Source: CAD feature listing. Evaluate the final solid. Frame: model axes, mm. Face numbers are marked on the shaded views. A direction names the side the tool comes from. Give positions to 0.01 mm unless a question says otherwise; leave off trailing zeros. Order: outer loops, then holes, each group sorted by start corner. A loop starts at its lowest first (then second) coordinate and runs counter-clockwise, first axis right, second up. Notation, with made-up numbers: (7.5, 28.25) -> (56.5, 28.25) arc R34 cw to (56.5, 60.25) -> close; hole circle Ø6 at (-23, -35). An arc over 180 degrees is marked (long way). Answer in a Markdown table with one row per item.
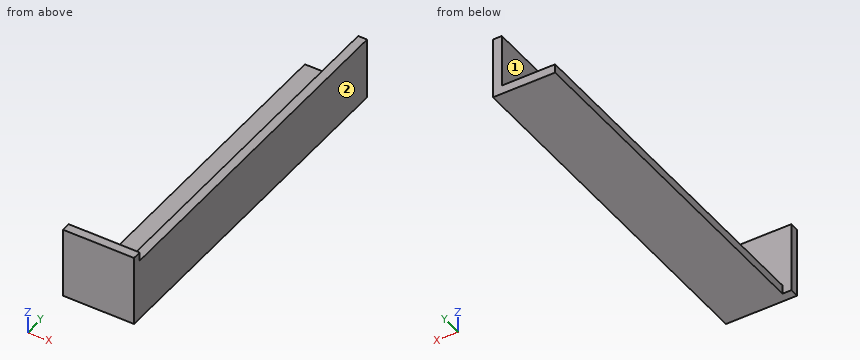
```python
from build123d import *

# Parameters (mm, degrees)
SKETCH_1_W           = 100
SKETCH_1_H           = 100
EXTRUDE_1_DEPTH      = 10
EXTRUDE_2_DEPTH      = 400
SKETCH_3_OUTSIDE_W   = 188.74
SKETCH_3_OUTSIDE_H   = 188.74
SKETCH_3_OUTSIDE_W_2 = 80
SKETCH_3_OUTSIDE_H_2 = 80
CUT_EXTRUDE_1_DEPTH  = 400


with BuildPart() as part:
    # 草图1 → 凸台-拉伸1 (new body)
    with BuildSketch(Plane(origin=(0, 0, 0), x_dir=(1, 0, 0), z_dir=(0, 1, 0))):
        with Locations((11.323542268, -6.987712791)):
            Rectangle(SKETCH_1_W, SKETCH_1_H)
    extrude(amount=EXTRUDE_1_DEPTH)

    # 草图2 → 凸台-拉伸2 (add)
    with BuildSketch(Plane(origin=(0, 10, 0), x_dir=(1, 0, 0), z_dir=(0, 1, 0))):
        Polygon((51.323542268, 33.012287209), (-18.676457732, 33.012287209), (-18.676457732, 23.012287209), (41.323542268, 23.012287209), (41.323542268, -36.987712791), (51.323542268, -36.987712791), align=None)
    extrude(amount=EXTRUDE_2_DEPTH)

    # 草图3 outside → 切除-拉伸1 (cut)
    with BuildSketch(Plane(origin=(0, 10, 0), x_dir=(1, 0, 0), z_dir=(0, 1, 0))):
        with Locations((11.324, -6.988)):
            Rectangle(SKETCH_3_OUTSIDE_W, SKETCH_3_OUTSIDE_H)
        with Locations((11.323542268, -6.987712791)):
            Rectangle(SKETCH_3_OUTSIDE_W_2, SKETCH_3_OUTSIDE_H_2, mode=Mode.SUBTRACT)
    extrude(amount=-CUT_EXTRUDE_1_DEPTH, mode=Mode.SUBTRACT)


solid = part.part
```
(1) Access query for the marked faces 1 and 2. Directions: +Z, -Z, +X, -X, +Y, -Y. A direction counts if a zero-diameter tool reaches every point of the face in a straight line with its end or side. Return the directions, or none.
A:
| item | result |
|---|---|
| face 1 | +Z, -X, +Y |
| face 2 | +Z, -Z, +X, +Y, -Y |
(2) First-contact query: pin 1 Ø5 at (x, y) = (13.5, 216.5) entering from +Z; pin 2 Ø1 at (x, z) = (-2, 14) entering from +Y; pin 3 Ø3 at (x, y) = (47.5, 126.5) entering from +Z. Flat tips, straight axial feed; report the tip coordinate or a pass-through.
A:
| item | result |
|---|---|
| pin 1 | stops at z = -23.01 |
| pin 2 | stops at y = 10 |
| pin 3 | stops at z = 36.99 |
(3) Section query A-A (z = 15.5). Return the cut outline in (x, y), plus the area to 3 significant figures.
A:
| item | result |
|---|---|
| outline | (-28.68, 0) -> (51.32, 0) -> (51.32, 410) -> (41.32, 410) -> (41.32, 10) -> (-28.68, 10) -> close |
| area | 4,800 mm^2 |
(4) Section query B-B (x = 36). Return the cut outline in (y, z).
A:
| item | result |
|---|---|
| outline | (0, -33.01) -> (410, -33.01) -> (410, -23.01) -> (10, -23.01) -> (10, 46.99) -> (0, 46.99) -> close |
(5) Ray query, probe 1 along Y at (x, z) = (5, -4); probe 2 along X at (y, z) = (171, -22); probe 3 along Z at (x, y) = (45, 364). Return the intervals inside material, ascending.
A:
| item | result |
|---|---|
| probe 1 | y = 0 to 10 |
| probe 2 | x = 41.32 to 51.32 |
| probe 3 | z = -33.01 to 36.99 |
